Verification items for the finished model (mm, model axes). Face numbers are marked on the shaded views. A direction names the side the tool comes from. Give positions to 0.01 mm unless a question says otherwise; leave off trailing zeros. Loops run counter-clockwise (first coordinate to the right, second up) from the corner with the lowest first, then second, coordinate; pieces in that order, holes last. Notation, with made-up numbers: (5, -1) - (28, -1) arc R14 cw to (28, 15) - close; hole circle Ø1 at (-36, -7.5). An arc over 180 degrees is marked (long way). One line per item, written item: value. Start each with the question number.
1. Sectioned sample at B-B (y = -373). Record the cut outline in (x, z) (3 decimals).
2. Gauge pin test, flat ends, axial feed: pin 1 (5 mm diameter, centred on x = 235.5, z = 19.5, fed in from +Y); pin 2 (6 mm diameter, centred on x = -135, y = -405.5, fed in from +Z); pin 3 (3 mm diameter, centred on x = 54, y = -375, fed in from -Z). Record the tip position at first contact, or that the pin passes through.
3. Mould release check, pull along X, two halves, no side actions. Record for the marked faces 1 and 2: pulls with the +X half, pulls with the -X half, needs draft (parallel to the pull), parting line crosses it, or undercut.
4. Sectioned sample at C-C (y = -626.5). Record the cut outline in (x, z), plus the area to 3 significant figures.
5. Access from +Z, -Z, +X, -X, +Y, -Y to the whole of each face (thin tool, end or side, straight path). Record for the marked faces 3 and 4.
6. Scan lines: L1, parallel to X at y = -816, z = 0 (3 decimals); L2, parallel to Z at x = 0, y = -363 (3 decimals). Record each from-to range of solid material in increasing order. Write a range as [from, to].
7. Sectioned sample at A-A (x = 0). Record the cut outline in (y, z) (3 decimals), plus the area to 3 significant figures.
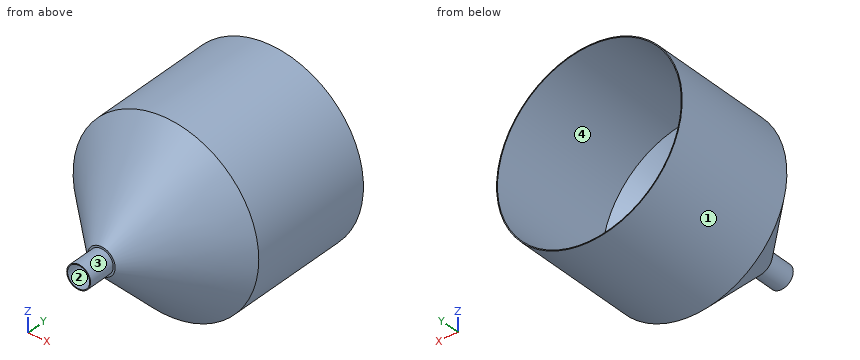
from build123d import *

# Parameters (mm, degrees)
CROQUIS1_R              = 334.8
SALIENTE_EXTRUIR1_DEPTH = 461.3
CROQUIS3_R              = 50
CROQUIS2_R              = 334.8
CROQUIS4_R              = 43
SALIENTE_EXTRUIR2_DEPTH = 100
VACIADO1_T              = -3.175


with BuildPart() as part:
    # Croquis1 → Saliente-Extruir1 (new body)
    with BuildSketch(Plane(origin=(0, 0, 0), x_dir=(1, 0, 0), z_dir=(0, 1, 0))):
        with Locations(Location((0, 0, 0), (0, 0, 270))):
            Circle(CROQUIS1_R)
    extrude(amount=-SALIENTE_EXTRUIR1_DEPTH)

    # Croquis3 → Recubrir1 section 0
    with BuildSketch(Plane(origin=(0, -746.1, 0), x_dir=(1, 0, 0), z_dir=(0, 1, 0))):
        Circle(CROQUIS3_R)
    # Croquis2 → Recubrir1 section 1
    with BuildSketch(Plane.XZ.offset(461.3)):
        Circle(CROQUIS2_R)
    loft()

    # Croquis4 → Saliente-Extruir2 (add)
    with BuildSketch(Plane.XZ.offset(746.1)):
        with Locations(Location((0, 0, 0), (0, 0, 270))):
            Circle(CROQUIS4_R)
    extrude(amount=SALIENTE_EXTRUIR2_DEPTH)

    # Vaciado1
    vaciado1_openings = [part.faces().sort_by_distance(p)[0] for p in [
        (0, -846.1, 0),
        (0, 0, 0),
    ]]
    offset(amount=VACIADO1_T, openings=vaciado1_openings, kind=Kind.INTERSECTION)


solid = part.part
Results are:
1. outline: circle Ø669.6 at (0, 0); hole circle Ø663.25 at (0, 0)
2. pin 1: stops at y = -552.8
2. pin 2: stops at z = 307.68
2. pin 3: stops at z = -330.66
3. face 1: parting line crosses it
3. face 2: undercut
4. outline: circle Ø339.2 at (0, 0); hole circle Ø330.22 at (0, 0)
4. area: 4,720 mm^2
5. face 3: -Y
5. face 4: +Y
6. L1: x = [-43, -39.825], [39.825, 43]
6. L2: z = [-334.8, -331.625], [331.625, 334.8]
7. outline: (-846.1, -43) - (-746.1, -43) - (-746.1, -50) - (-461.3, -334.8) - (0, -334.8) - (0, -331.625) - (-459.985, -331.625) - (-742.925, -48.685) - (-742.925, -39.825) - (-846.1, -39.825) - close; (-846.1, 39.825) - (-742.925, 39.825) - (-742.925, 48.685) - (-459.985, 331.625) - (0, 331.625) - (0, 334.8) - (-461.3, 334.8) - (-746.1, 50) - (-746.1, 43) - (-846.1, 43) - close
7. area: 6,170 mm^2
